Source: CAD feature listing. Evaluate the final solid. Frame: model axes, mm. A direction names the side the tool comes from. Round coordinates to 2 decimals unless told otherwise and drop trailing zeros. Order: outer loops, then holes, each group sorted by start corner. A loop starts at its lowest first (then second) coordinate and runs counter-clockwise, first axis right, second up. Notation, with made-up numbers: (-21.75, 64.25) - (-3.75, 64.25) arc R23 cw to (-3.75, 97.25) - close; hole circle Ø9 at (40, -3). An arc over 180 degrees is marked (long way). Use one line per item in the form item = value. Start each with the question number.
Q1. Cut plane A-A, the plane x = 44.45. Return the cut outline in (y, z) (3 decimals).
Q2. Cut plane B-B, the plane z = 1.5. Give the number of separate pieces and of enclosed holes in the cut face, and give its area (3 significant figures).
Q3. Set-up query: faces 1 (the flat face through (68, -15.875, 2)), 2 (the flat face through (-1, -57.15, 2)). Return all of +Z, -Z, +X, -X, +Y, -Y with unobstructed straight access to the full face (end or side cutting, diameter ignored); none if empty.
Q4. Ray query, line 1 (Y direction, x = -17.78, z = 1.4); line 2 (X direction, y = 44.45, z = 1.45); line 3 (X direction, y = 43, z = 1.3). Return the intervals inside material, ascending. Write a range as [from, to].
Q5. Draft query along X for faces 3 (the cylindrical face through (70.56, 42.553, 1.565)), 4 (the cylindrical face through (44.488, 19.675, 1.61)), 5 (the flat face through (-1, 1, 0)), 6 (the flat face through (-88.9, -1, 2)). Return one class per face: released by +X, released by -X, zero draft, split by the parting line, or undercut.
Q6. Pin query (flat end, axial travel): pin 1 Ø2 at (x, y) = (39.37, -53.34) entering from -Z. Return the tip coordinate at first contact, or that it passes through.
from build123d import *

# Parameters (mm, degrees)
SKETCH1_W                      = 177.8
SKETCH1_H                      = 114.3
BOSS_EXTRUDE1_DEPTH            = 3.175
SKETCH8_R                      = 2
CUT_EXTRUDE2_DEPTH             = 106.732743864
SKETCH9_R                      = 1.27
CUT_EXTRUDE3_DEPTH             = 106.732743864
LPATTERN1_COUNT                = 2
LPATTERN1_PITCH                = 57.15
SKETCH10_R                     = 1.27
CUT_EXTRUDE4_DEPTH             = 106.732743864
SKETCH11_R                     = 1.75
CUT_EXTRUDE5_DEPTH             = 106.732743864
F_6_CLEARANCE_HOLE1_AT_2_COUNT = 2
F_6_CLEARANCE_HOLE1_AT_2_PITCH = 88.9
CUT_EXTRUDE6_DEPTH             = 106.732743864


with BuildPart() as part:
    # Sketch1 → Boss-Extrude1 (new body)
    with BuildSketch(Plane.XY):
        Rectangle(SKETCH1_W, SKETCH1_H)
    extrude(amount=BOSS_EXTRUDE1_DEPTH)

    # Sketch8 → Cut-Extrude2 (cut, through all)
    with BuildSketch(Plane.XY.offset(3.175)):
        with Locations((-79.375, 28.575)):
            Circle(SKETCH8_R)
        with Locations((15.875, 28.575)):
            Circle(SKETCH8_R)
        with Locations((15.875, -22.225)):
            Circle(SKETCH8_R)
        with Locations((-79.375, -22.225)):
            Circle(SKETCH8_R)
    extrude(amount=-CUT_EXTRUDE2_DEPTH, mode=Mode.SUBTRACT)

    # Sketch9 → Cut-Extrude3 (cut, through all)
    with BuildSketch(Plane.XY.offset(3.175)):
        with Locations((-63.5, -35.56)):
            Circle(SKETCH9_R)
        with Locations((-17.78, -35.56)):
            Circle(SKETCH9_R)
        with Locations((-17.78, -53.34)):
            Circle(SKETCH9_R)
        with Locations((-63.5, -53.34)):
            Circle(SKETCH9_R)
    cut_extrude3 = extrude(amount=-CUT_EXTRUDE3_DEPTH, mode=Mode.SUBTRACT)

    # LPattern1: Cut-Extrude3 ×2
    with Locations(*[(i * LPATTERN1_PITCH, 0, 0) for i in range(1, LPATTERN1_COUNT)]):
        add(cut_extrude3, mode=Mode.SUBTRACT)

    # Sketch10 → Cut-Extrude4 (cut, through all)
    with BuildSketch(Plane.XY.offset(3.175)):
        with Locations((35.56, 52.705)):
            Circle(SKETCH10_R)
        with Locations((53.34, 52.705)):
            Circle(SKETCH10_R)
        with Locations((53.34, 34.925)):
            Circle(SKETCH10_R)
        with Locations((35.56, 34.925)):
            Circle(SKETCH10_R)
    extrude(amount=-CUT_EXTRUDE4_DEPTH, mode=Mode.SUBTRACT)

    # Sketch11 → Cut-Extrude5 (cut, through all)
    with BuildSketch(Plane.XY.offset(3.175)):
        with Locations((44.45, -25.4)):
            Circle(SKETCH11_R)
        with BuildLine():
            Line((42.7, 21.425), (42.7, 27.775))
            ThreePointArc((42.7, 27.775), (44.45, 29.525), (46.2, 27.775))
            Line((46.2, 27.775), (46.2, 21.425))
            ThreePointArc((46.2, 21.425), (44.45, 19.675), (42.7, 21.425))
        make_face()
    extrude(amount=-CUT_EXTRUDE5_DEPTH, mode=Mode.SUBTRACT)

    # Sketch15 → #6 Clearance Hole1 (revolve, cut)
    with BuildSketch(Plane(origin=(70.64375, 44.45, 0), x_dir=(0, 1, 0), z_dir=(1, 0, 0))):
        Polygon((0, 0), (0, 26.540824014), (1.89865, 25.4), (1.89865, 0), align=None)
    f_6_clearance_hole1 = revolve(axis=Axis((70.64375, 44.45, -6.35), (0, 0, 1)), mode=Mode.SUBTRACT)

    # #6 Clearance Hole1 at 2: #6 Clearance Hole1 ×2
    with Locations(*[(0, -i * F_6_CLEARANCE_HOLE1_AT_2_PITCH, 0) for i in range(1, F_6_CLEARANCE_HOLE1_AT_2_COUNT)]):
        add(f_6_clearance_hole1, mode=Mode.SUBTRACT)

    # Sketch16 → Cut-Extrude6 (cut, through all)
    with BuildSketch(Plane(origin=(0, 0, 0), x_dir=(-1, 0, 0), z_dir=(0, 0, -1))):
        with BuildLine():
            Line((-74.295, 22.225), (-61.595, 22.225))
            ThreePointArc((-61.595, 22.225), (-58.42, 19.05), (-61.595, 15.875))
            Line((-61.595, 15.875), (-74.295, 15.875))
            ThreePointArc((-74.295, 15.875), (-77.47, 19.05), (-74.295, 22.225))
        make_face()
    cut_extrude6 = extrude(amount=-CUT_EXTRUDE6_DEPTH, mode=Mode.SUBTRACT)

    # Mirror4: Cut-Extrude6 across plane
    add(cut_extrude6.mirror(Plane.ZX), mode=Mode.SUBTRACT)

    # Mirror5: #6 Clearance Hole1 across plane
    add(f_6_clearance_hole1.mirror(Plane(origin=(0, 0, 0), x_dir=(0, 0, 1), z_dir=(1, 0, 0))), mode=Mode.SUBTRACT)

    # Mirror5 copy 1 sketch → Mirror5 copy 1 (revolve, cut)
    with BuildSketch(Plane(origin=(-70.64375, -44.45, 0), x_dir=(0, 1, 0), z_dir=(-1, 0, 0))):
        Polygon((0, 0), (0, -26.540824014), (1.89865, -25.4), (1.89865, 0), align=None)
    revolve(axis=Axis((-70.64375, -44.45, -6.35), (0, 0, -1)), mode=Mode.SUBTRACT)


solid = part.part
Completed:
q1.outline = (-57.15, 0) - (-27.15, 0) - (-27.15, 3.175) - (-57.15, 3.175) - close; (-23.65, 0) - (19.675, 0) - (19.675, 3.175) - (-23.65, 3.175) - close; (29.525, 0) - (57.15, 0) - (57.15, 3.175) - (29.525, 3.175) - close
q2.separate_pieces = 1
q2.enclosed_holes = 24
q2.area = 19,900 mm2
q3.face_1 = +Z, -Z
q3.face_2 = +Z, -Z, +X, -X, -Y
q4.line_1 = [-57.15, -54.61], [-52.07, -36.83], [-34.29, 57.15]
q4.line_2 = [-88.9, -72.54], [-68.75, 68.75], [72.54, 88.9]
q4.line_3 = [-88.9, -71.87], [-69.42, 69.42], [71.87, 88.9]
q5.face_3 = undercut
q5.face_4 = undercut
q5.face_5 = zero draft
q5.face_6 = released by -X
q6.pin_1 = through
